Here's how the part is built. I have some questions about the finished solid (model axes, mm). Face numbers are marked on the shaded views. A direction names the side the tool comes from. Give positions to 0.01 mm unless a question says otherwise; leave off trailing zeros. Order: outer loops, then holes, each group sorted by start corner. A loop starts at its lowest first (then second) coordinate and runs counter-clockwise, first axis right, second up. Notation, with made-up numbers: M 74,80 L 131,80 A30 ccw 131,108 Z; hole C -16.75,72 d6. An arc over 180 degrees is marked long. Use CSV: the item, a comma, the result in double quotes. Start each with the question number.
```python
from build123d import *

# Parameters (mm, degrees)
SKETCH1_W           = 70.993
SKETCH1_H           = 31.115
BOSS_EXTRUDE1_DEPTH = 18.415
SKETCH2_R           = 1.905
SKETCH2_W           = 7.62
SKETCH2_H           = 6.35
BOSS_EXTRUDE2_DEPTH = 6.35
SKETCH3_R           = 5.715
CUT_EXTRUDE1_DEPTH  = 2.54


with BuildPart() as part:
    # Sketch1 → Boss-Extrude1 (new body)
    with BuildSketch(Plane.XY):
        with Locations((35.4965, 15.5575)):
            Rectangle(SKETCH1_W, SKETCH1_H)
    extrude(amount=BOSS_EXTRUDE1_DEPTH)

    # Sketch2 → Boss-Extrude2 (add)
    with BuildSketch(Plane.XY.offset(18.415)):
        with Locations(Location((57.023, 10.794999954, 0), (0, 0, 180))):
            Circle(SKETCH2_R)
        with Locations((27.94, 15.5575)):
            Rectangle(SKETCH2_W, SKETCH2_H)
    extrude(amount=BOSS_EXTRUDE2_DEPTH)

    # Sketch3 → Cut-Extrude1 (cut)
    with BuildSketch(Plane(origin=(0, 0, 0), x_dir=(-1, 0, 0), z_dir=(0, 0, -1))):
        with Locations((-19.05, 15.5575)):
            Circle(SKETCH3_R)
    extrude(amount=-CUT_EXTRUDE1_DEPTH, mode=Mode.SUBTRACT)


solid = part.part
```
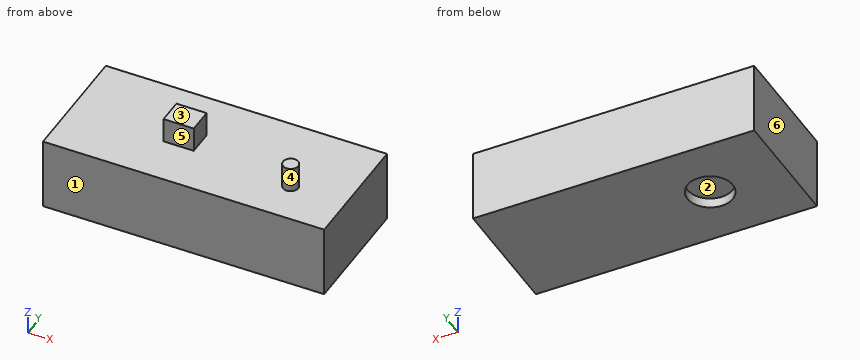
Q1. Imagine slicing it at B-B, the plane y = 25.5. Please give me the cut outline in (x, z) (3 decimals).
Q2. For the marked faces 5 and 6, which set-ups out of +Z, -Z, +X, -X, +Y, -Y let a thin tool reach every point of the face, with its end or its side?
Q3. I need wall thicknesses on line 1 (Y direction, x = 19.05, z = 0.75) (1 decimal); line 2 (Z direction, x = 24.5, y = 4.5) (3 decimals). Which ranges of each line are inside material? Lowest first, please. Write a range as [from, to].
Q4. Imagine slicing it at D-D, the plane x = 60.5. Please give me the cut outline in (y, z) (3 decimals), then the cut area to 3 significant figures.
Q5. Imagine slicing it at A-A, the plane x = 19.05. Please give me the cut outline in (y, z) (1 decimal), then the cut area to 3 significant figures.
Q6. We'd pull the mould along Y, two halves only. Please class the marked faces 1, 2, 3 and 4: pulls with the +Y half, pulls with the -Y half, needs draft (parallel to the pull), parting line crosses it, or undercut.
Q7. For P1, Ø3, axis at x = 26.5, z = 22, coming from the -Y side; P2, Ø5, axis at x = 27.5, z = 18.5, coming from the +Y side (3 decimals); P3, Ø1.5, axis at x = 37.5, y = 26, coming from the +Z side (3 decimals); P4, Ø3.5, axis at x = 18, y = 17.5, coming from the -Z side, each with a flat end and sliding along its axis, tell me the tip position at first contact or that it passes through.
Reply:
1,outline,"M 0,0 L 70.993,0 L 70.993,18.415 L 0,18.415 Z"
2,face 5,"+Z, -X, -Y"
2,face 6,"+Z, -Z, -X, +Y, -Y"
3,line 1,"y = [0, 9.8], [21.3, 31.1]"
3,line 2,"z = [0, 18.415]"
4,outline,"M 0,0 L 31.115,0 L 31.115,18.415 L 0,18.415 Z"
4,area,"573 mm^2"
5,outline,"M 0,0 L 9.8,0 L 9.8,2.5 L 21.3,2.5 L 21.3,0 L 31.1,0 L 31.1,18.4 L 0,18.4 Z"
5,area,"544 mm^2"
6,face 1,"pulls with the -Y half"
6,face 2,"undercut"
6,face 3,"needs draft"
6,face 4,"parting line crosses it"
7,P1,"stops at y = 12.38"
7,P2,"stops at y = 31.115"
7,P3,"stops at z = 18.415"
7,P4,"stops at z = 2.54"
